Geometry check sheet. Reference: the model listing, model coordinates, mm. A direction names the side the tool comes from. Give positions to 0.01 mm unless a question says otherwise; leave off trailing zeros. Loops run counter-clockwise (first coordinate to the right, second up) from the corner with the lowest first, then second, coordinate; pieces in that order, holes last. Notation, with made-up numbers: (38, 13.25) -> (95, 13.25) arc R20 ccw to (95, 18.25) -> close; hole circle Ø5 at (28.25, -2.75). An arc over 180 degrees is marked (long way). Write item = value, one per line.
Autodesk Inventor part; units mm, degrees
ref_plane "YZ Plane" through (0, 0, 0) normal (1, 0, 0) x (0, 1, 0)
ref_plane "XZ Plane" through (0, 0, 0) normal (0, 1, 0) x (-1, 0, 0)
ref_plane "XY Plane" through (0, 0, 0) normal (0, 0, 1) x (1, 0, 0)
sketch "Sketch1" plane through (0, 0, 0) normal (0, 0, 1) x (1, 0, 0)
  line L0 (4.5085, 2.54) -> (4.5085, -2.54)
  line L1 (4.5085, -2.54) -> (7.6835, -2.54)
  line L2 (7.6835, -2.54) -> (7.6835, -0.9525)
  line L3 (7.6835, -0.9525) -> (6.096, -0.9525)
  line L4 (6.096, -0.9525) -> (6.096, 0.9525)
  line L5 (6.096, 0.9525) -> (7.6835, 0.9525)
  line L6 (7.6835, 0.9525) -> (7.6835, 2.54)
  line L7 (7.6835, 2.54) -> (4.5085, 2.54)
  line L8 (0, 0) -> (0, 2.54) construction
  point P0 (4.5085, 0)
  point P1 (6.096, 0)
  dimension "d0" = 6.096
  dimension "d1" = 1.905
  dimension "d2" = 5.08
  dimension "d3" = 1.5875
  dimension "d4" = 1.5875
  dimension "d5" = 1.5875
revolve "Revolution1" add sketch "Sketch1" angle 360 about axis through (0, 0, 0) along (0, 1, 0)
fillet "Fillet1" radius 0.3969 4 edges at (-7.6835, -0.9525, 0) (-7.6835, -2.54, 0) (-7.6835, 0.9525, 0) (-7.6835, 2.54, 0)
chamfer "Chamfer1" distance 0.7937 angle 45 1 edges at (-6.096, 0.9525, 0) measured on face at (6.7601, 0.9525, 1.0676)
equation "\"d4\" = d3"
properties part number ".5 tpu grommet" material "Rubber, Black"
Item 1: Section check C-C, the plane y = 0.5. Record the cut outline in (x, z).
Answer:
outline = circle Ø12.87 at (0, 0); hole circle Ø9.02 at (0, 0)
Item 2: Thickness scan on L1, parallel to Z at x = 0, y = -0.35; L2, parallel to X at y = 1.4, z = 0; L3, parallel to Y at x = 3.25, z = 6.5. Record the ranges inside material, lowest first. Write a range as [from, to].
Answer:
L1 = [-6.1, -4.51], [4.51, 6.1]
L2 = [-7.68, -4.51], [4.51, 7.68]
L3 = [-2.54, -0.95], [0.95, 2.54]
Item 3: Draft check along Y on faces 3 (the flat face through (0, 2.54, 5)), 4 (the flat face through (0, -2.54, 5)), 5 (the cylindrical face through (-0.794, -0.389, -6.044)), 6 (the cylindrical face through (7.33, 1.75, -2.31)). Enter one of: +Y half, -Y half, draft (parallel to the pull), parting line (faces both ways), or undercut.
Answer:
face_3 = +Y half
face_4 = -Y half
face_5 = undercut
face_6 = draft
Item 4: Tool access check on faces 1 (the flat face through (-2, -0.952, 6)), 2 (the cylindrical face through (-0.98, -0.04, -4.4)). Record the directions out of +Z, -Z, +X, -X, +Y, -Y that give a thin tool (end or side, any length) a straight path to the whole face; none if there is none.
Answer:
face_1 = none
face_2 = +Y, -Y
Item 5: Gauge pin test, flat ends, axial feed: pin 1 (2 mm diameter, centred on x = 4, y = 0.5, fed in from +Z); pin 2 (7.5 mm diameter, centred on x = -3.5, z = -2, fed in from +Y); pin 3 (1.5 mm diameter, centred on x = 6, y = 1.5, fed in from +Z); pin 4 (2 mm diameter, centred on y = 0.5, z = -1, fed in from -X). Record the tip position at first contact, or that the pin passes through.
Answer:
pin_1 = 6.91
pin_2 = 2.54
pin_3 = 5.61
pin_4 = -7.67
Item 6: Section check B-B, the plane z = 0. Record the cut outline in (x, y).
Answer:
outline = (-7.68, -2.14) arc R0.4 ccw to (-7.29, -2.54) -> (-4.51, -2.54) -> (-4.51, 2.54) -> (-7.29, 2.54) arc R0.4 ccw to (-7.68, 2.14) -> (-7.68, 1.35) arc R0.4 ccw to (-7.29, 0.95) -> (-6.89, 0.95) -> (-6.1, 0.16) -> (-6.1, -0.95) -> (-7.29, -0.95) arc R0.4 ccw to (-7.68, -1.35) -> close; (4.51, -2.54) -> (7.29, -2.54) arc R0.4 ccw to (7.68, -2.14) -> (7.68, -1.35) arc R0.4 ccw to (7.29, -0.95) -> (6.1, -0.95) -> (6.1, 0.16) -> (6.89, 0.95) -> (7.29, 0.95) arc R0.4 ccw to (7.68, 1.35) -> (7.68, 2.14) arc R0.4 ccw to (7.29, 2.54) -> (4.51, 2.54) -> close
Item 7: Section check A-A, the plane x = 0. Record the cut outline in (y, z).
Answer:
outline = (-2.54, -7.29) arc R0.4 ccw to (-2.14, -7.68) -> (-1.35, -7.68) arc R0.4 ccw to (-0.95, -7.29) -> (-0.95, -6.1) -> (0.16, -6.1) -> (0.95, -6.89) -> (0.95, -7.29) arc R0.4 ccw to (1.35, -7.68) -> (2.14, -7.68) arc R0.4 ccw to (2.54, -7.29) -> (2.54, -4.51) -> (-2.54, -4.51) -> close; (-2.54, 4.51) -> (2.54, 4.51) -> (2.54, 7.29) arc R0.4 ccw to (2.14, 7.68) -> (1.35, 7.68) arc R0.4 ccw to (0.95, 7.29) -> (0.95, 6.89) -> (0.16, 6.1) -> (-0.95, 6.1) -> (-0.95, 7.29) arc R0.4 ccw to (-1.35, 7.68) -> (-2.14, 7.68) arc R0.4 ccw to (-2.54, 7.29) -> close
